Geometry: final body of the model. Coordinates: model frame, mm. Face numbers are marked on the shaded views. A direction names the side the tool comes from. Coordinates: 2 decimals unless noted, no trailing zeros. Write each loop counter-clockwise with the first axis right and the second up, starting at its lowest first coordinate (ties: lowest second). Pieces come first, ordered by that corner, then holes.
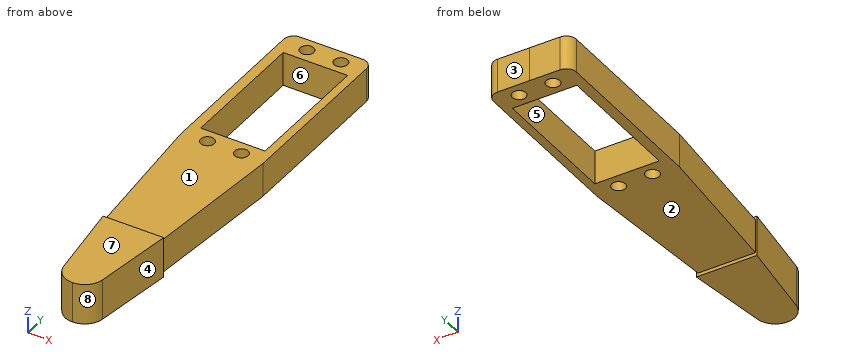
from build123d import *

# Parameters (mm, degrees)
BOSS_EXTRU_1_DEPTH           = 10
ESQUISSE2_W                  = 19
ESQUISSE2_H                  = 39
ENL_V_MAT_EXTRU_1_DEPTH      = 14
ENL_V_MAT_EXTRU_2_DEPTH      = 15
ENL_V_MAT_EXTRU_2_DEPTH_BACK = 7
ESQUISSE3_R                  = 2
CONG_1_R                     = 3
CONG_2_R                     = 3
BOSS_EXTRU_4_DEPTH           = 1
BOSS_EXTRU_4_DEPTH_BACK      = 11
CONG_4_R                     = 5.755572


with BuildPart() as part:
    # Esquisse1 → Boss.-Extru.1 (new body)
    with BuildSketch(Plane.XY):
        Polygon((-0.581785688, 80.233199881), (11.918214312, 80.233199881), (11.918214312, 28.233199881), (8.257673117, -13.606977439), (7.257673726, -13.608081293), (3.5, -40.345319149), (0, -40.345319149), (-3.826627386, -40.353406678), (-7.643319911, -13.624529819), (-8.643319302, -13.625633672), (-12.396222382, 28.206360286), (-12.511023087, 80.206233562), align=None)
    extrude(amount=BOSS_EXTRU_1_DEPTH)

    # Esquisse2 → Enlèv. mat.-Extru.1 (cut)
    with BuildSketch(Plane.XY.offset(10)):
        with Locations((0, 52.733199881)):
            Rectangle(ESQUISSE2_W, ESQUISSE2_H)
    extrude(amount=-ENL_V_MAT_EXTRU_1_DEPTH, mode=Mode.SUBTRACT)

    # Esquisse3 → Enlèv. mat.-Extru.2 (cut, two sides: drawn at the far end of the back side and taken through both)
    with BuildSketch(Plane.XY.offset(-ENL_V_MAT_EXTRU_2_DEPTH_BACK)):
        with Locations((5, 76.233199881)):
            Circle(ESQUISSE3_R)
        with Locations((5, 29.233199881)):
            Circle(ESQUISSE3_R)
        with Locations((-5, 29.233199881)):
            Circle(ESQUISSE3_R)
        with Locations((-5, 76.233199881)):
            Circle(ESQUISSE3_R)
    extrude(amount=ENL_V_MAT_EXTRU_2_DEPTH + ENL_V_MAT_EXTRU_2_DEPTH_BACK, mode=Mode.SUBTRACT)

    # Congé1
    cong_1_edges = [part.edges().sort_by_distance(p)[0] for p in [
        (11.918214312, 80.233199881, 5),
    ]]
    fillet(cong_1_edges, radius=CONG_1_R)

    # Congé2
    cong_2_edges = [part.edges().sort_by_distance(p)[0] for p in [
        (-12.511023087, 80.206233562, 5),
    ]]
    fillet(cong_2_edges, radius=CONG_2_R)

    # Esquisse4 → Boss.-Extru.4 (add, two sides: drawn at the far end of the back side and taken through both)
    with BuildSketch(Plane(origin=(0, 0, 0), x_dir=(-1, 0, 0), z_dir=(0, 0, -1)).offset(-BOSS_EXTRU_4_DEPTH_BACK)):
        Polygon((-8.792588162, -13.607529366), (9.080964972, -13.607529366), (5.141727933, -42.4046649), (-4.912145705, -42.4046649), align=None)
    extrude(amount=BOSS_EXTRU_4_DEPTH + BOSS_EXTRU_4_DEPTH_BACK)

    # Congé4
    cong_4_edges = [part.edges().sort_by_distance(p)[0] for p in [
        (4.912145705, -42.4046649, 5),
        (-5.141727933, -42.4046649, 5),
    ]]
    fillet(cong_4_edges, radius=CONG_4_R - 0.0001)  # a hair under: the kernel refuses the full size


solid = part.part
Item 1: Section C-C, the plane z = 6.75. State how many separate pieces and enclosed holes the cut face has, plus the area to 3 significant figures.
Derived:
separate pieces: 1
enclosed holes: 5
area: 1,730 mm2
Item 2: Section B-B, the plane y = 49. Output: boundary loops of the cut face in (x, z), plus the area to 3 significant figures.
Derived:
outline: (-12.44, 0) - (-9.5, 0) - (-9.5, 10) - (-12.44, 10) - close; (9.5, 0) - (11.92, 0) - (11.92, 10) - (9.5, 10) - close
area: 53.6 mm2
Item 3: Pin query (flat end, axial travel): pin 1 (5 mm diameter, centred on x = -5, y = 29.23, fed in from -Z); pin 2 (10 mm diameter, centred on x = 6, y = -8.5, fed in from +Z); pin 3 (2 mm diameter, centred on x = -9, z = 4.5, fed in from +Y); pin 4 (3.5 mm diameter, centred on x = 5, y = 29.23, fed in from -Z). Return the tip coordinate at first contact, or that it passes through.
Derived:
pin 1: stops at z = 0
pin 2: stops at z = 10
pin 3: stops at y = 80.22
pin 4: passes through
Item 4: Section D-D, the plane y = 9. Output: boundary loops of the cut face in (x, z).
Derived:
outline: (-10.67, 0) - (10.24, 0) - (10.24, 10) - (-10.67, 10) - close
Item 5: Material intervals for probe 1 along Y at (x, z) = (5, 3.75); probe 2 along Y at (x, z) = (-5, 6); probe 3 along X at (y, z) = (35, 9), sorted ascending.
Derived:
probe 1: y = -39.28 to 27.23, 31.23 to 33.23, 72.23 to 74.23, 78.23 to 80.23
probe 2: y = -39.7 to 27.23, 31.23 to 33.23, 72.23 to 74.23, 78.23 to 80.22
probe 3: x = -12.41 to -9.5, 9.5 to 11.92
Item 6: Section A-A, the plane x = 1.5. Output: boundary loops of the cut face in (y, z).
Derived:
outline: (-42.17, -1) - (-13.61, -1) - (-13.61, 0) - (33.23, 0) - (33.23, 10) - (-13.61, 10) - (-13.61, 11) - (-42.17, 11) - close; (72.23, 0) - (80.23, 0) - (80.23, 10) - (72.23, 10) - close
Item 7: Set-up query: the marked faces 1, 2, 3, 4 and 5. Return all of +Z, -Z, +X, -X, +Y, -Y with unobstructed straight access to the full face (end or side cutting, diameter ignored); none if empty.
Derived:
face 1: +Z, +X, -X, +Y
face 2: -Z, +X, -X, +Y
face 3: +Z, -Z, +X, -X, +Y
face 4: +Z, -Z, +X, -Y
face 5: +Z, -Z
Item 8: Pull-direction query (Y, two-part tool) for the marked faces 6, 7 and 8; classes: released by +Y, released by -Y, zero draft, split by the parting line, or undercut.
Derived:
face 6: undercut
face 7: zero draft
face 8: released by -Y
